from build123d import *

# Parameters (mm, degrees)
CROQUIS1_R                 = 4
SALIENTE_EXTRUIR1_DEPTH    = 3
CROQUIS2_W                 = 40
CROQUIS2_H                 = 665
CROQUIS2_R                 = 12.7
SALIENTE_EXTRUIR2_DEPTH    = 20
CORTAR_EXTRUIR1_DEPTH      = 99
CORTAR_EXTRUIR1_DEPTH_BACK = 71
CROQUIS3_R                 = 4


with BuildPart() as part:
    # Croquis1 → Saliente-Extruir1 (new body)
    with BuildSketch(Plane.XY):
        with BuildLine():
            Line((-50, 85), (50, 85))
            ThreePointArc((50, 85), (71.213203436, 76.213203436), (80, 55))
            Line((80, 55), (80, -55))
            ThreePointArc((80, -55), (71.213203436, -76.213203436), (50, -85))
            Line((50, -85), (-50, -85))
            ThreePointArc((-50, -85), (-71.213203436, -76.213203436), (-80, -55))
            Line((-80, -55), (-80, 55))
            ThreePointArc((-80, 55), (-71.213203436, 76.213203436), (-50, 85))
        make_face()
        with Locations((0, 70.6)):
            Circle(CROQUIS1_R, mode=Mode.SUBTRACT)
        with Locations((0, -70.6)):
            Circle(CROQUIS1_R, mode=Mode.SUBTRACT)
        with Locations((-30, 70.6)):
            Circle(CROQUIS1_R, mode=Mode.SUBTRACT)
        with Locations((30, 70.6)):
            Circle(CROQUIS1_R, mode=Mode.SUBTRACT)
        with Locations((-30, -70.6)):
            Circle(CROQUIS1_R, mode=Mode.SUBTRACT)
        with Locations((30, -70.6)):
            Circle(CROQUIS1_R, mode=Mode.SUBTRACT)
    extrude(amount=SALIENTE_EXTRUIR1_DEPTH)

    # Croquis2 → Saliente-Extruir2 (add)
    with BuildSketch(Plane.XY):
        with Locations((0, -332.5)):
            Rectangle(CROQUIS2_W, CROQUIS2_H)
        with Locations((0, -247.75)):
            Circle(CROQUIS2_R, mode=Mode.SUBTRACT)
    extrude(amount=-SALIENTE_EXTRUIR2_DEPTH)

    # Croquis3 → Cortar-Extruir1 (cut, two sides: drawn at the far end of the back side and taken through both)
    with BuildSketch(Plane.XY.offset(-CORTAR_EXTRUIR1_DEPTH_BACK)):
        with Locations((0, -70.6)):
            Circle(CROQUIS3_R)
    extrude(amount=CORTAR_EXTRUIR1_DEPTH + CORTAR_EXTRUIR1_DEPTH_BACK, mode=Mode.SUBTRACT)


solid = part.part
Source: CAD feature listing. Evaluate the final solid. Frame: model axes, mm. A direction names the side the tool comes from. Give positions to 0.01 mm unless a question says otherwise; leave off trailing zeros. Order: outer loops, then holes, each group sorted by start corner. A loop starts at its lowest first (then second) coordinate and runs counter-clockwise, first axis right, second up. Notation, with made-up numbers: (56, 56.5) -> (66, 56.5) arc R7 ccw to (66, 69.5) -> close; hole circle Ø10 at (62, 7.5). An arc over 180 degrees is marked (long way). Use a Markdown table: item, result.
1) Section query D-D, the plane x = -64. Return the cut outline in (y, z).
Answer list:
| item | result |
|---|---|
| outline | (-81.53, 0) -> (81.53, 0) -> (81.53, 3) -> (-81.53, 3) -> close |
2) Mould query, pull axis Y, two halves, no side actions, for faces 3 (the flat face through (0, -371, 0)), 4 (the cylindrical face through (-2.75, -260.15, -9.86)), 5 (the flat face through (0, -665, -10)). Classes: +Y half, -Y half, draft (parallel to the pull), parting line (faces both ways), or undercut.
Answer list:
| item | result |
|---|---|
| face 3 | draft |
| face 4 | undercut |
| face 5 | -Y half |
3) Reachability of faces 1 (the cylindrical face through (70.979, 76.445, 1.479)), 2 (the flat face through (0, 0, -10)) from +Z, -Z, +X, -X, +Y, -Y: full face, straight path, thin tool, end or side. Return the list, or none.
Answer list:
| item | result |
|---|---|
| face 1 | +Z, -Z, +X, +Y |
| face 2 | -Z, +X, -X, +Y |
4) Section query B-B, the plane z = -16.5. Return the cut outline in (x, y), then the cut area to 3 significant figures.
Answer list:
| item | result |
|---|---|
| outline | (-20, -665) -> (20, -665) -> (20, 0) -> (-20, 0) -> close; hole circle Ø25.4 at (0, -247.75); hole circle Ø8 at (0, -70.6) |
| area | 26,000 mm² |
5) Section query A-A, the plane y = -247.75. Return the cut outline in (x, z), then the cut area to 3 significant figures.
Answer list:
| item | result |
|---|---|
| outline | (-20, -20) -> (-12.7, -20) -> (-12.7, 0) -> (-20, 0) -> close; (12.7, -20) -> (20, -20) -> (20, 0) -> (12.7, 0) -> close |
| area | 292 mm² |
6) Section query C-C, the plane y = -356.5. Return the cut outline in (x, z), then the cut area to 3 significant figures.
Answer list:
| item | result |
|---|---|
| outline | (-20, -20) -> (20, -20) -> (20, 0) -> (-20, 0) -> close |
| area | 800 mm² |
7) Contact query for flat-ended pins moving along their axis: P1, Ø2.5, axis at x = 18, z = 2, coming from the -Y side; P2, Ø10.5, axis at x = 30, y = 70.6, coming from the -Z side; P3, Ø10, axis at y = -295, z = -8.5, coming from the +X side. Output: stop coordinate, or through.
Answer list:
| item | result |
|---|---|
| P1 | y = -85 |
| P2 | z = 0 |
| P3 | x = 20 |
8) Ray query, line 1 along Y through (x, z) = (30, 0.85); line 2 along Y through (x, z) = (0, -13.5); line 3 along X through (y, z) = (-70.6, -8.5). Return the intervals inside material, ascending. Write a range as [from, to].
Answer list:
| item | result |
|---|---|
| line 1 | [-85, -74.6], [-66.6, 66.6], [74.6, 85] |
| line 2 | [-665, -260.45], [-235.05, -74.6], [-66.6, 0] |
| line 3 | [-20, -4], [4, 20] |
